Can you work these out from the drawing? Everything is in mm from the part's minimum corner. A direction names the side the tool comes from. Give positions to 0.01 mm unless a question says otherwise; leave off trailing zeros. Write each loop counter-clockwise with the first axis right and the second up, starting at its lowest first coordinate (ties: lowest second). Pieces come first, ordered by that corner, then holes. Notation, with made-up numbers: (-32, 5) -> (9, 5) arc R11 cw to (9, 16) -> close; hole circle Ø2 at (67.25, 52). An arc over 180 degrees is marked (long way). Use one line per item in the form item = value.
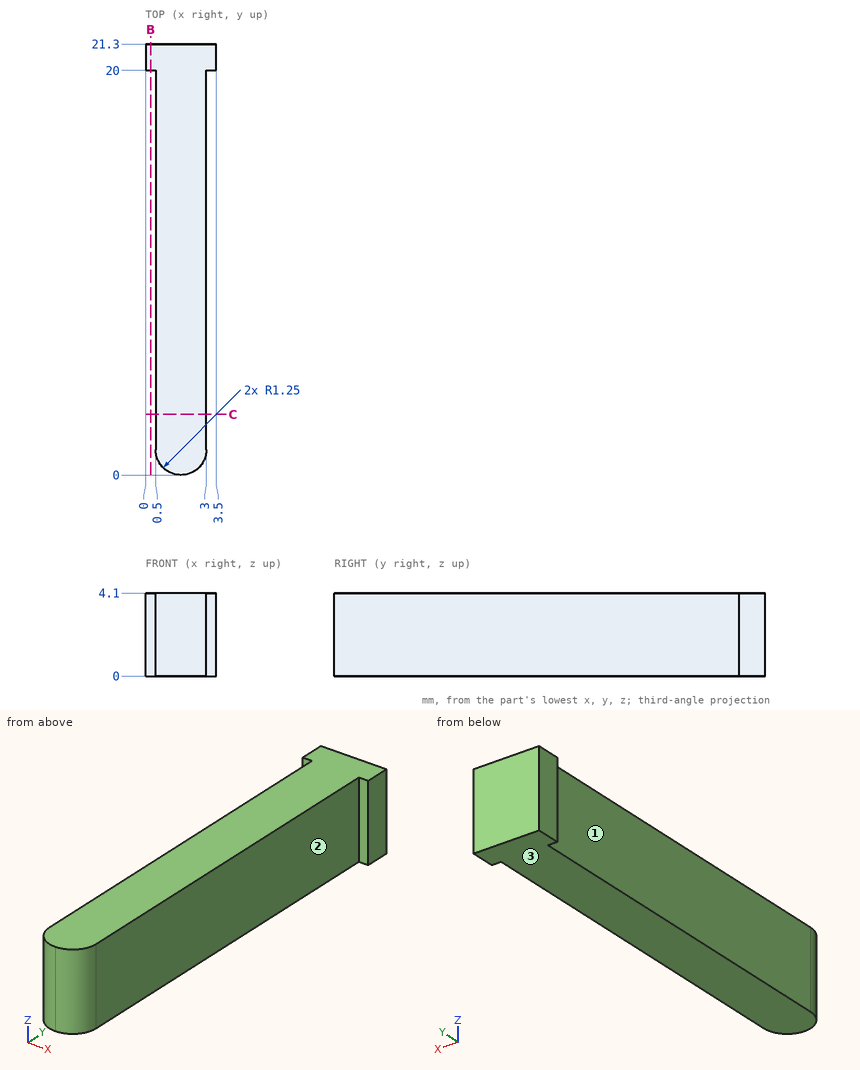
Q1. If I drill on line 1 along Y through (x, z) = (3.05, 2.85); line 2 along X through (y, z) = (8.5, 1.1); line 3 along Y through (x, z) = (0.65, 2.95) (1 decimal), over which ranges is the centre line in solid material (lowest first)? Write a range as from..to.
Result set:
line_1 = 20..21.3
line_2 = 0.5..3
line_3 = 0.7..21.3
Q2. Will these pins go through, and if not, where does the flat tip stop? pin 1 Ø1.5 at (y, z) = (4.5, 1.5) entering from -X; pin 2 Ø2 at (y, z) = (10.5, 2) entering from +X.
Result set:
pin_1 = 0.5
pin_2 = 3
Q3. I want a section at C-C, the plane y = 3. Write out the boundary of the cut face in (x, z).
Result set:
outline = (0.5, 0) -> (3, 0) -> (3, 4.1) -> (0.5, 4.1) -> close
Q4. Which directions (+Z, -Z, +X, -X, +Y, -Y) give clear straight access to the entire face, cutting with the end or side of a thin tool? Please do the marked faces 1, 2 and 3.
Result set:
face_1 = +Z, -Z, -X, -Y
face_2 = +Z, -Z, +X, -Y
face_3 = -Z, +X, -X, +Y, -Y
Q5. I want a section at B-B, the plane x = 0.25. Write out the boundary of the cut face in (y, z).
Result set:
outline = (20, 0) -> (21.3, 0) -> (21.3, 4.1) -> (20, 4.1) -> close
